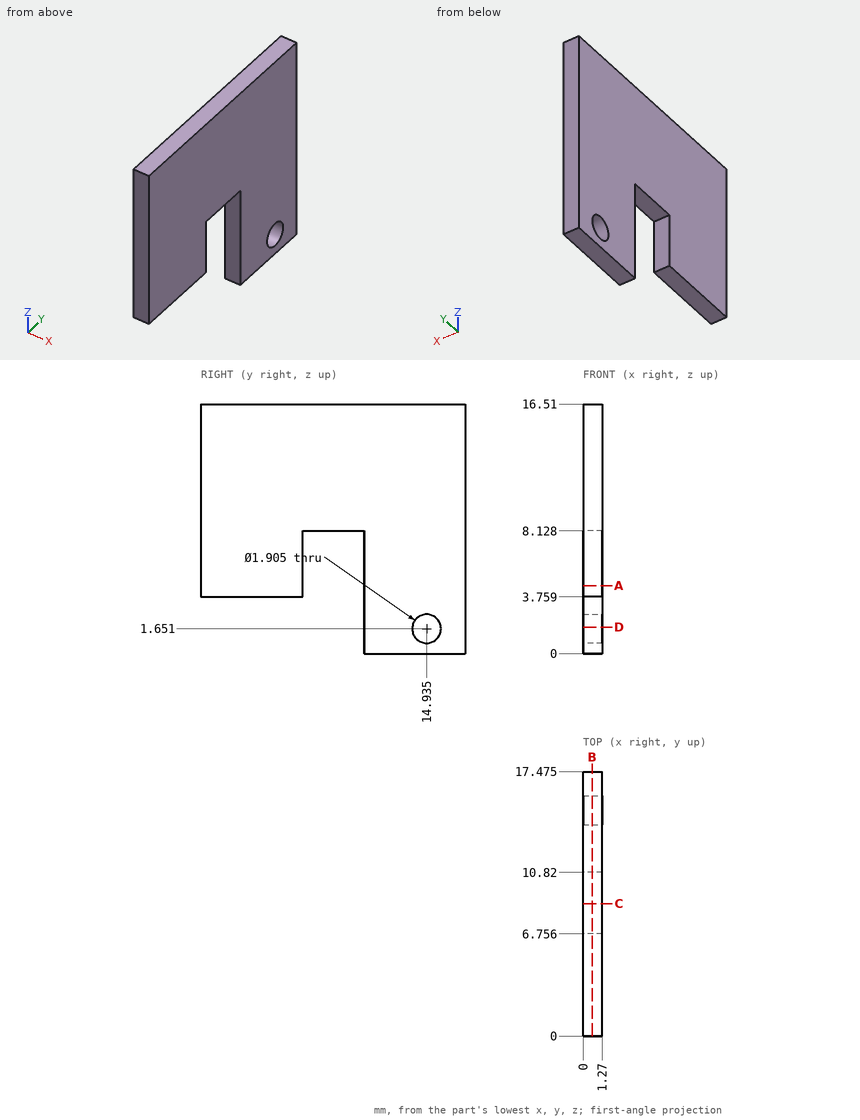
For this review, use the dimensioned drawing (mm, ordinates from the lowest corner) and the shaded views. Round coordinates to 2 decimals unless told otherwise and drop trailing zeros. Order: outer loops, then holes, each group sorted by start corner. A loop starts at its lowest first (then second) coordinate and runs counter-clockwise, first axis right, second up.
1) For L1, parallel to Y at x = 0.85, z = 5.25 (1 decimal); L2, parallel to Z at x = 0.95, y = 7.5; L3, parallel to Z at x = 0.45, y = 5.25, list the stretches that pass through material, from the lowest coordinate up.
The answers:
L1: y = 0 to 6.8, 10.8 to 17.5
L2: z = 8.13 to 16.51
L3: z = 3.76 to 16.51
2) Consider section B-B (x = 0.6). State the section outline as (y, z) points (1 decimal), plus the area to 3 significant figures.
The answers:
outline: (0, 3.8) - (6.8, 3.8) - (6.8, 8.1) - (10.8, 8.1) - (10.8, 0) - (17.5, 0) - (17.5, 16.5) - (0, 16.5) - close; hole circle Ø1.9 at (14.9, 1.7)
area: 227 mm2
3) Consider section D-D (z = 1.75). State the section outline as (x, y) points (1 decimal).
The answers:
outline: (0, 10.8) - (1.3, 10.8) - (1.3, 14) - (0, 14) - close; (0, 15.9) - (1.3, 15.9) - (1.3, 17.5) - (0, 17.5) - close
4) Consider section C-C (y = 8.75). State the section outline as (x, z) points.
The answers:
outline: (0, 8.13) - (1.27, 8.13) - (1.27, 16.51) - (0, 16.51) - close
5) Consider section A-A (z = 4.5). State the section outline as (x, y) points (1 decimal).
The answers:
outline: (0, 0) - (1.3, 0) - (1.3, 6.8) - (0, 6.8) - close; (0, 10.8) - (1.3, 10.8) - (1.3, 17.5) - (0, 17.5) - close
